from build123d import *

# Parameters (mm, degrees)
F0_W     = 233
F0_H     = 81
F0_W_2   = 227.4
F0_H_2   = 75.4
F1_DEPTH = 8.8
F2_W     = 10
F2_H     = 4.4
F3_DEPTH = 25
F4_W     = 10
F4_H     = 1.2
F5_DEPTH = 2.4
F6_R     = 10
F7_DEPTH = 0.6


with BuildPart() as f1:
    # F0 (on Top) → F1 (new body)
    with BuildSketch(Plane.XY):
        Rectangle(F0_W, F0_H)
        Rectangle(F0_W_2, F0_H_2, mode=Mode.SUBTRACT)
    extrude(amount=F1_DEPTH)

    # F2 (on face) → F3 (cut)
    with BuildSketch(Plane(origin=(0, 40.5, 0), x_dir=(-1, 0, 0), z_dir=(0, 1, 0))):
        with Locations((76.5, 2.2)):
            Rectangle(F2_W, F2_H)
    extrude(amount=-F3_DEPTH, mode=Mode.SUBTRACT)

    # F4 (on face) → F5 (cut)
    with BuildSketch(Plane(origin=(0, 0, 4.4), x_dir=(1, 0, 0), z_dir=(0, 0, -1))):
        with Locations((-76.5, -38.3)):
            Rectangle(F4_W, F4_H)
    extrude(amount=-F5_DEPTH, mode=Mode.SUBTRACT)

    # F6 (on face) → F7 (join)
    with BuildSketch(Plane.XY.offset(8.8)):
        with Locations((-116.5, 40.5)):
            Circle(F6_R)
        with Locations((-116.5, -40.5)):
            Circle(F6_R)
        with Locations((116.5, -40.5)):
            Circle(F6_R)
        with Locations((116.5, 40.5)):
            Circle(F6_R)
    extrude(amount=-F7_DEPTH)


solid = f1.part
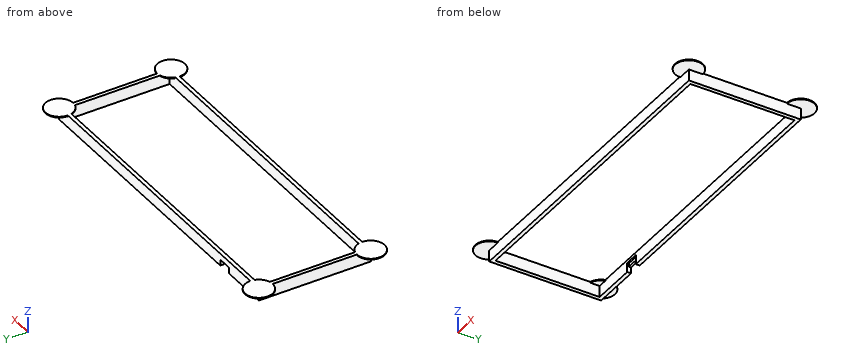
Design review of the part built by this model. Coordinates are the model's own, in mm. Round coordinates to 2 decimals unless told otherwise and drop trailing zeros. Write each loop counter-clockwise with the first axis right and the second up, starting at its lowest first coordinate (ties: lowest second). Pieces come first, ordered by that corner, then holes. Notation, with made-up numbers: M 80.5,76.25 L 131.5,76.25 A18 ccw 131.5,94.25 Z; hole C 42,-32.75 d3. An arc over 180 degrees is marked long. One line per item, written item: value. Start each with the question number.
1. Clearance check with flat-ended pins moving along their axes: P1, Ø2.5, axis at y = -15, z = 2, coming from the -X side; P2, Ø0.7, axis at x = -78.5, z = 6, coming from the -Y side; P3, Ø1.4, axis at y = 39, z = 2, coming from the +X side. State where each tip first meets the part, or that it passes through.
2. Take a section at B-B on x = 57. State the section outline as (y, z) points.
3. To check wall thickness, follow probe 1 along X at (y, z) = (-13.5, 5); probe 2 along Y at (x, z) = (-94, 2.75); probe 3 along X at (y, z) = (-39, 3.5). State the ranges of each line that lie inside material, in increasing order. Write a range as from..to.
4. Take a section at A-A on y = 13.5. State the section outline as (x, z) points, then the cut area to 3 significant figures.
Computed:
1. P1: stops at x = -116.5
1. P2: stops at y = -40.5
1. P3: stops at x = 116.5
2. outline: M -40.5,0 L -37.7,0 L -37.7,8.8 L -40.5,8.8 Z; M 37.7,0 L 40.5,0 L 40.5,8.8 L 37.7,8.8 Z
3. probe 1: x = -116.5..-113.7, 113.7..116.5
3. probe 2: y = -40.5..-37.7, 37.7..40.5
3. probe 3: x = -116.5..116.5
4. outline: M -116.5,0 L -113.7,0 L -113.7,8.8 L -116.5,8.8 Z; M 113.7,0 L 116.5,0 L 116.5,8.8 L 113.7,8.8 Z
4. area: 49.3 mm²
